Can you work these out from the model? Positions are in its coordinate system, mm. Face numbers are marked on the shaded views. A direction names the side the tool comes from. Coordinates: 2 decimals unless noted, no trailing zeros. Order: outer loops, then holes, each group sorted by start corner. A loop starts at its lowest first (then second) coordinate and runs counter-clockwise, first axis right, second up. Notation, with made-up numbers: M 37,-8.75 L 59,-8.75 A23 ccw 59,19.25 Z; hole C 74,56.25 d4. An arc over 180 degrees is marked long. Answer as a JSON object with one key per item and string values.
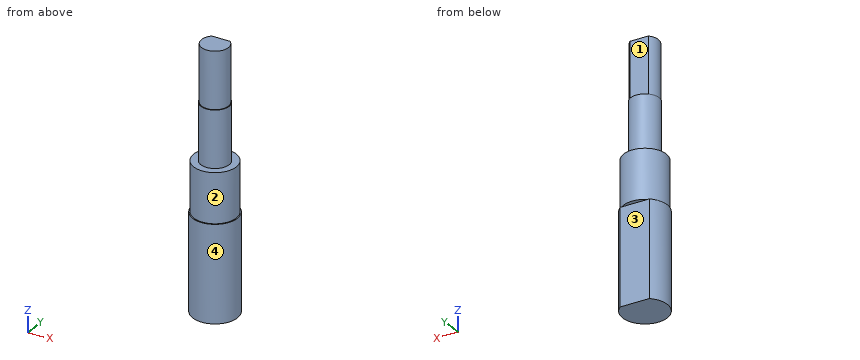
from build123d import *

# Parameters (mm, degrees)
SKETCH1_R           = 5
BOSS_EXTRUDE1_DEPTH = 21.637500032
SKETCH2_R           = 4.7625
BOSS_EXTRUDE2_DEPTH = 11.1125
SKETCH3_R           = 3.175
BOSS_EXTRUDE3_DEPTH = 12.7
SKETCH4_W           = 25.4
SKETCH4_H           = 2.38125
CUT_EXTRUDE1_DEPTH  = 21.637500032
SKETCH6_R           = 3
BOSS_EXTRUDE4_DEPTH = 12.7
SKETCH7_W           = 25.37250579
SKETCH7_H           = 1.5875
CUT_EXTRUDE3_DEPTH  = 12.7


with BuildPart() as part:
    # Sketch1 → Boss-Extrude1 (new body)
    with BuildSketch(Plane.XY):
        Circle(SKETCH1_R)
    extrude(amount=BOSS_EXTRUDE1_DEPTH)

    # Sketch2 → Boss-Extrude2 (add)
    with BuildSketch(Plane.XY.offset(21.637500032)):
        Circle(SKETCH2_R)
    extrude(amount=BOSS_EXTRUDE2_DEPTH)

    # Sketch3 → Boss-Extrude3 (add)
    with BuildSketch(Plane.XY.offset(32.750000032)):
        Circle(SKETCH3_R)
    extrude(amount=BOSS_EXTRUDE3_DEPTH)

    # Sketch4 → Cut-Extrude1 (cut)
    with BuildSketch(Plane(origin=(0, 0, 0), x_dir=(-1, 0, 0), z_dir=(0, 0, -1))):
        with Locations((0, 5)):
            Rectangle(SKETCH4_W, SKETCH4_H)
    extrude(amount=-CUT_EXTRUDE1_DEPTH, mode=Mode.SUBTRACT)

    # Sketch6 → Boss-Extrude4 (add)
    with BuildSketch(Plane.XY.offset(45.450000032)):
        Circle(SKETCH6_R)
    extrude(amount=BOSS_EXTRUDE4_DEPTH)

    # Sketch7 → Cut-Extrude3 (cut)
    with BuildSketch(Plane.XY.offset(58.150000032)):
        with Locations((0, 3)):
            Rectangle(SKETCH7_W, SKETCH7_H)
    extrude(amount=-CUT_EXTRUDE3_DEPTH, mode=Mode.SUBTRACT)


solid = part.part
Item 1: Please list where these lines run through material, in increasing order: line 1 (Z direction, x = -3, y = -1.75); line 2 (X direction, y = 0, z = 33) (3 decimals); line 3 (X direction, y = 0, z = 31.5).
Answers follow:
{"line 1": "z = 0 to 32.75", "line 2": "x = -3.175 to 3.175", "line 3": "x = -4.76 to 4.76"}
Item 2: Which directions (+Z, -Z, +X, -X, +Y, -Y) give clear straight access to the entire face, cutting with the end or side of a thin tool? Please do the marked faces 1, 2, 3 and 4.
Answers follow:
{"face 1": "+Z, +X, -X, +Y", "face 2": "+Z", "face 3": "-Z, +X, -X, +Y", "face 4": "+Z, -Z"}
Item 3: I'm going to push flat-ended pins straight in: pin 1 (1 mm diameter, centred on x = -3, z = 36.5, fed in from -Y); pin 2 (1 mm diameter, centred on x = -0.5, y = 4.5, fed in from -Z); pin 3 (5 mm diameter, centred on x = 3, z = 17.5, fed in from +Y). Where does each tip first touch, or does it pass through?
Answers follow:
{"pin 1": "stops at y = -1.96", "pin 2": "stops at z = 21.64", "pin 3": "stops at y = 3.81"}
Item 4: I want a section at C-C, the plane z = 19.5. Write out the boundary of the cut face in (x, y), plus the area to 3 significant figures.
Answers follow:
{"outline": "M -3.24,3.81 A5 ccw long 3.24,3.81 Z", "area": "73.3 mm^2"}
Item 5: I want a section at D-D, the plane y = -3.75. Write out the boundary of the cut face in (x, z).
Answers follow:
{"outline": "M -3.31,0 L 3.31,0 L 3.31,21.64 L 2.94,21.64 L 2.94,32.75 L -2.94,32.75 L -2.94,21.64 L -3.31,21.64 Z"}
